Autodesk Inventor part; units mm, degrees
sketch "Sketch2" plane through (0, 0, 0) normal (1, 0, 0) x (0, 1, 0)
  line L0 (50, 50) -> (-50, 50)
  line L1 (-50, 50) -> (-50, -50)
  line L2 (-50, -50) -> (50, -50)
  line L3 (50, -50) -> (50, 50)
  line L4 (-70, 0) -> (70, 0)
  line L5 (0, 70) -> (0, -70)
  point P0 (0, 0)
  point P1 (50, 0)
  point P2 (0, 50)
  dimension "d0" = 100
  dimension "d1" = 100
extrude "Extrusion1" add sketch "Sketch2" along normal mid plane 10
sketch "Sketch3" plane through (5, 0, 0) normal (1, 0, 0) x (0, 0, -1)
  line L0 (-47, 47) -> (47, 47)
  line L1 (47, 47) -> (47, -47)
  line L2 (47, -47) -> (-47, -47)
  line L3 (-47, -47) -> (-47, 47)
  line L4 (0, -70) -> (0, 70)
  line L5 (-70, 0) -> (70, 0)
  point P0 (0, 0)
  point P1 (0, 47)
  point P2 (-47, 0)
  dimension "d4" = 94
  dimension "d5" = 94
extrude "Extrusion2" cut sketch "Sketch3" against normal blind 7
sketch "Sketch5" plane through (-5, 50, 50) normal (0, 1, 0) x (1, 0, 0)
  circle A0 centre (5, 5) radius 2.5
  line L0 (10, 0) -> (0, 0)
  line L1 (5, 120) -> (5, -20)
  circle A1 centre (5, 25) radius 2.5
  circle A2 centre (5, 45) radius 2.5
  circle A3 centre (5, 95) radius 2.5
  line L2 (0, 100) -> (10, 100)
  circle A4 centre (5, 75) radius 2.5
  circle A5 centre (5, 55) radius 2.5
  point P0 (5, 50)
  dimension "d26" = 5
  dimension "d27" = 5
  dimension "d30" = 20
  dimension "d35" = 5
  dimension "d36" = 5
  dimension "d39" = 20
extrude "Extrusion3" cut sketch "Sketch5" against normal blind 7
sketch "Sketch6" plane through (-5, -50, -50) normal (0, -1, 0) x (1, 0, 0)
  circle A0 centre (5, 95) radius 2.5
  line L0 (0, 100) -> (10, 100)
  line L1 (5, -20) -> (5, 120)
  line L2 (5, 120) -> (5, -20)
  line L3 (0, 0) -> (10, 0)
  line L4 (-2, 50) -> (12, 50)
  circle A1 centre (5, 5) radius 2.5
  point P0 (5, 50)
  dimension "d46" = 5
  dimension "d47" = 5
extrude "Extrusion4" add sketch "Sketch6" along normal blind 5
properties part number "Wall"
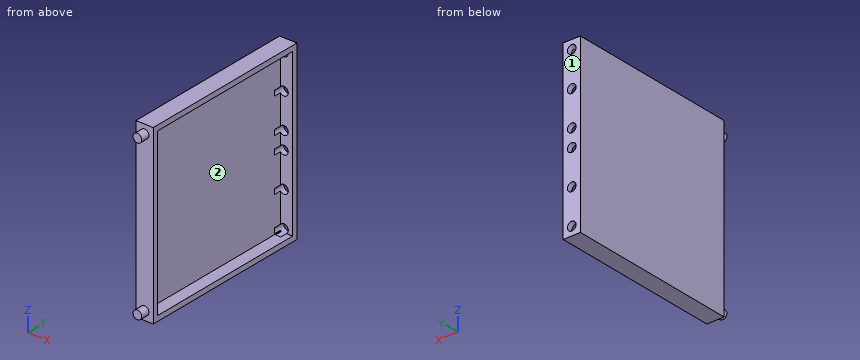
The listing builds one solid part. Answer for the finished solid, in the listing's coordinates (mm). Face numbers are marked on the shaded views. Coordinates: 2 decimals unless noted, no trailing zeros. Write each loop counter-clockwise with the first axis right and the second up, starting at its lowest first coordinate (ties: lowest second). Pieces come first, ordered by that corner, then holes. Notation, with made-up numbers: (33, 69.5) - (65, 69.5) arc R13 cw to (65, 92.5) - close; hole circle Ø1 at (0.5, 59). An arc over 180 degrees is marked (long way). One line per item, written item: value.
1) Consider line 1 along Z through (x, y) = (3.25, 5.5); line 2 along Z through (x, y) = (0, 46.5). Determine where each line is inside the solid, lowest interval first. Write a range as from..to.
Geometry check:
line 1: z = -50..-47, 47..50
line 2: z = -50..-47.5, 47.5..50
2) For a pull along Z with two mould halves and no side action, classify the marked faces 1 and 2 as pulls with the +Z half, pulls with the -Z half, needs draft (parallel to the pull), parting line crosses it, or undercut.
Geometry check:
face 1: needs draft
face 2: undercut
3) Each of these flat-tipped pins is pushed along its axis until it touches: pin 1 Ø0.6 at (x, z) = (-2, 5) entering from +Y; pin 2 Ø5.5 at (x, z) = (0, -3.5) entering from +Y; pin 3 Ø12 at (y, z) = (24, -12) entering from +X; pin 4 Ø5 at (x, z) = (2.5, -4.5) entering from -Y. Where does it stop, or does it pass through?
Geometry check:
pin 1: stops at y = 43
pin 2: stops at y = 50
pin 3: stops at x = -2
pin 4: stops at y = -50
4) Find section A-A (z = 25). Give the vertices of the cut face in (x, y), and give its area (3 significant figures).
Geometry check:
outline: (-5, -50) - (5, -50) - (5, -47) - (-2, -47) - (-2, 43) - (-2.5, 43) - (-2.5, 50) - (-5, 50) - close; (2.5, 47) - (5, 47) - (5, 50) - (2.5, 50) - close
area: 325 mm2
5) Find section D-D (x = -3.75). Give the vertices of the cut face in (y, z).
Geometry check:
outline: (-50, -50) - (50, -50) - (50, 50) - (-50, 50) - close
6) Find section B-B (y = -10.5). Give the vertices of the cut face in (x, z).
Geometry check:
outline: (-5, -50) - (5, -50) - (5, -47) - (-2, -47) - (-2, 47) - (5, 47) - (5, 50) - (-5, 50) - close
